The drawing under review shows one solid part. Ordinate dimensions are in mm from its lowest x, y, z. A direction names the side the tool comes from. Coordinates: 2 decimals unless noted, no trailing zeros. Loops run counter-clockwise (first coordinate to the right, second up) from the corner with the lowest first, then second, coordinate; pieces in that order, holes last. Notation, with made-up numbers: M -6,-18.75 L 8,-18.75 A30 ccw 8,9.25 Z; hole C -7,44 d9. An arc over 180 degrees is marked long. Return JSON: item names as keys, results as strings.
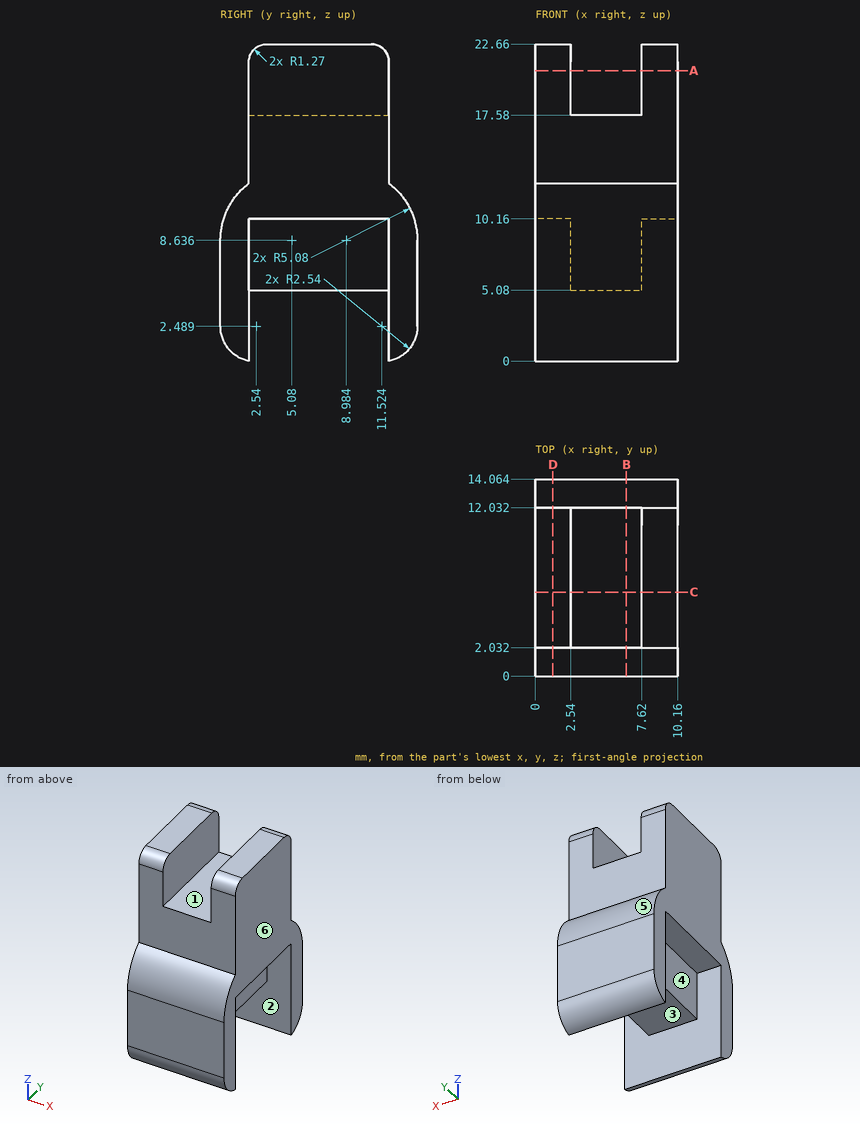
1. Add section B-B on x = 6.5. Give the boundary of the cut face in (y, z), plus the area to 3 significant figures.
Check values:
{"outline": "M 0,2.49 A2.54 ccw 2.03,0 L 2.03,5.08 L 12.03,5.08 L 12.03,0 A2.54 ccw 14.06,2.49 L 14.06,8.64 A5.08 ccw 12.03,12.7 L 12.03,17.58 L 2.03,17.58 L 2.03,12.7 A5.08 ccw 0,8.64 Z", "area": "169 mm²"}
2. Machinability: for the marked faces 1, 2 and 3, which of the approach directions +Z, -Z, +X, -X, +Y, -Y give a long, thin tool a straight path to every point of the face, cutting with its end or side? Answer none if there is none.
Check values:
{"face 1": "+Z, +Y, -Y", "face 2": "-Z", "face 3": "-Z, +X, -X"}
3. Add section A-A on z = 20.75. Give the boundary of the cut face in (x, y), plus the area to 3 significant figures.
Check values:
{"outline": "M 0,2.03 L 2.54,2.03 L 2.54,12.03 L 0,12.03 Z; M 7.62,2.03 L 10.16,2.03 L 10.16,12.03 L 7.62,12.03 Z", "area": "50.8 mm²"}
4. To check wall thickness, follow line 1 (Y direction, x = 7.25, z = 4.5); line 2 (X direction, y = 2.75, z = 19.5); line 3 (Z direction, x = 7.25, y = 5). State the ranges of each line that lie inside material, in increasing order.
Check values:
{"line 1": "0 to 2.03, 12.03 to 14.06", "line 2": "0 to 2.54, 7.62 to 10.16", "line 3": "5.08 to 17.58"}
5. Insertion check: pin 1 Ø1.3 at (x, y) = (9, 6.5) entering from -Z; pin 2 Ø1.5 at (x, y) = (7, 5.5) entering from -Z; pin 3 Ø6 at (x, z) = (2, 14) entering from +Y. Each pin has a flat end and moves straight along its axis. Give the tip position at first contact, or say it passes through.
Check values:
{"pin 1": "z = 10.16", "pin 2": "z = 5.08", "pin 3": "y = 13.48"}
6. The part is to be moulded in two halves that separate along Y. For the marked faces 4, 5 and 6, say which applies: released by +Y, released by -Y, zero draft, split by the parting line, or undercut.
Check values:
{"face 4": "undercut", "face 5": "released by +Y", "face 6": "zero draft"}
7. Add section C-C on y = 6. Give the boundary of the cut face in (x, z), plus the area to 3 significant figures.
Check values:
{"outline": "M 0,10.16 L 2.54,10.16 L 2.54,5.08 L 7.62,5.08 L 7.62,10.16 L 10.16,10.16 L 10.16,22.66 L 7.62,22.66 L 7.62,17.58 L 2.54,17.58 L 2.54,22.66 L 0,22.66 Z", "area": "127 mm²"}
8. Add section D-D on x = 1.25. Give the boundary of the cut face in (y, z), plus the area to 3 significant figures.
Check values:
{"outline": "M 0,2.49 A2.54 ccw 2.03,0 L 2.03,10.16 L 12.03,10.16 L 12.03,0 A2.54 ccw 14.06,2.49 L 14.06,8.64 A5.08 ccw 12.03,12.7 L 12.03,21.39 A1.27 ccw 10.76,22.66 L 3.3,22.66 A1.27 ccw 2.03,21.39 L 2.03,12.7 A5.08 ccw 0,8.64 Z", "area": "168 mm²"}
